```python
from build123d import *

# Parameters (mm, degrees)
SKETCH1_W           = 170
SKETCH1_H           = 145
BOSS_EXTRUDE1_DEPTH = 5
SKETCH2_W           = 150.6
SKETCH2_H           = 125.6
SKETCH2_W_2         = 144.4
SKETCH2_H_2         = 119.4
CUT_EXTRUDE1_DEPTH  = 2.5
SKETCH5_W           = 71
SKETCH5_H           = 7.5
SKETCH5_W_2         = 8
SKETCH5_H_2         = 25
BOSS_EXTRUDE2_DEPTH = 17.5
SKETCH6_W           = 2.5
SKETCH6_H           = 7.5
SKETCH6_H_2         = 25
BOSS_EXTRUDE3_DEPTH = 21.5
SKETCH7_W           = 71
SKETCH7_H           = 2.5
BOSS_EXTRUDE4_DEPTH = 4
BOSS_EXTRUDE6_DEPTH = 21.5


with BuildPart() as part:
    # Sketch1 → Boss-Extrude1 (new body)
    with BuildSketch(Plane(origin=(0, 0, 0), x_dir=(1, 0, 0), z_dir=(0, 1, 0))):
        Rectangle(SKETCH1_W, SKETCH1_H)
    extrude(amount=BOSS_EXTRUDE1_DEPTH)

    # Sketch2 → Cut-Extrude1 (cut)
    with BuildSketch(Plane(origin=(0, 5, 0), x_dir=(1, 0, 0), z_dir=(0, 1, 0))):
        Rectangle(SKETCH2_W, SKETCH2_H)
        Rectangle(SKETCH2_W_2, SKETCH2_H_2, mode=Mode.SUBTRACT)
    extrude(amount=-CUT_EXTRUDE1_DEPTH, mode=Mode.SUBTRACT)

    # Sketch5 → Boss-Extrude2 (add)
    with BuildSketch(Plane(origin=(0, 5, 0), x_dir=(1, 0, 0), z_dir=(0, 1, 0))):
        with Locations((0, 29.05)):
            Rectangle(SKETCH5_W, SKETCH5_H)
        with Locations((-31.5, -47.2)):
            Rectangle(SKETCH5_W_2, SKETCH5_H_2)
        with Locations((31.5, -47.2)):
            Rectangle(SKETCH5_W_2, SKETCH5_H_2)
    extrude(amount=BOSS_EXTRUDE2_DEPTH)

    # Sketch6 → Boss-Extrude3 (add)
    with BuildSketch(Plane(origin=(0, 5, 0), x_dir=(1, 0, 0), z_dir=(0, 1, 0))):
        with Locations((36.75, 29.05)):
            Rectangle(SKETCH6_W, SKETCH6_H)
        with Locations((-36.75, 29.05)):
            Rectangle(SKETCH6_W, SKETCH6_H)
        with Locations((36.75, -47.2)):
            Rectangle(SKETCH6_W, SKETCH6_H_2)
        with Locations((-36.75, -47.2)):
            Rectangle(SKETCH6_W, SKETCH6_H_2)
    extrude(amount=BOSS_EXTRUDE3_DEPTH)

    # Sketch7 → Boss-Extrude4 (add)
    with BuildSketch(Plane(origin=(0, 22.5, 0), x_dir=(1, 0, 0), z_dir=(0, 1, 0))):
        with Locations((0, 31.55)):
            Rectangle(SKETCH7_W, SKETCH7_H)
    extrude(amount=BOSS_EXTRUDE4_DEPTH)

    # Sketch9 → Boss-Extrude6 (add)
    with BuildSketch(Plane(origin=(0, 5, 0), x_dir=(1, 0, 0), z_dir=(0, 1, 0))):
        Polygon((38, -59.7), (72.2, -59.7), (72.2, -57.8), (72.2, 57.8), (72.2, 59.7), (-72.2, 59.7), (-72.2, 57.8), (-72.2, -57.8), (-72.2, -59.7), (-38, -59.7), (-38, -57.2), (-69.7, -57.8), (-69.7, 57.8), (69.7, 57.8), (69.7, -57.2), (38, -57.2), align=None)
    extrude(amount=BOSS_EXTRUDE6_DEPTH)


solid = part.part
```
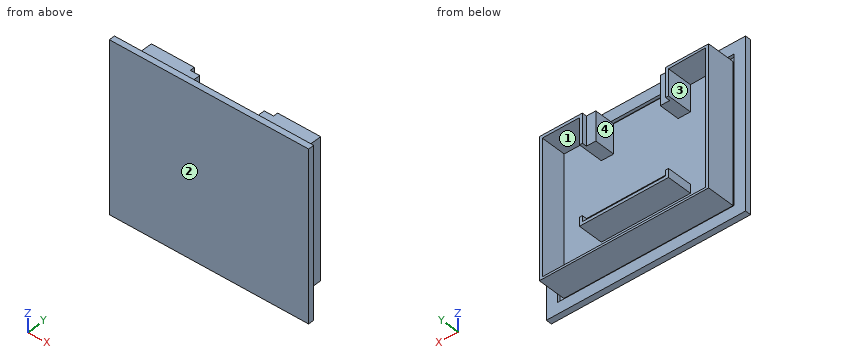
Check sheet for the modelled part. Datum: model origin and axes. Units: mm. Face numbers are marked on the shaded views. A direction names the side the tool comes from. Give positions to 0.01 mm unless a question says otherwise; leave off trailing zeros. Loops run counter-clockwise (first coordinate to the right, second up) from the corner with the lowest first, then second, coordinate; pieces in that order, holes last. Notation, with made-up numbers: (11, -21.5) - (32, -21.5) arc R21 ccw to (32, 3.5) - close; hole circle Ø11 at (-28.75, -11.75). An arc over 180 degrees is marked (long way). One line per question, with ' | ' between items. Start each with the question number.
1. Cross-section at A-A, the plane y = 18.25. Enter the section's corners in (x, z).
2. Material ranges on line 1 along Z through (x, y) = (-54.5, 2.75); line 2 along X through (y, z) = (5.5, 47); line 3 along Z through (x, y) = (14.5, 18.75), recorded low to high. Write a range as [from, to].
3. Cross-section at B-B, the plane z = 43.5. Enter the section's corners in (x, y).
4. Cross-section at D-D, the plane z = -52. Enter the section's corners in (x, y).
5. Cross-section at C-C, the plane x = 46.5. Enter the section's corners in (y, z), plus the area to 3 significant figures.
6. Draft check along Z on the marked faces 3 and 4. Enter one of: released by +Z, released by -Z, zero draft, split by the parting line, or undercut.
7. Gauge pin test, flat ends, axial feed: pin 1 Ø8 at (x, y) = (-12.5, 15) entering from +Z; pin 2 Ø14 at (y, z) = (13.5, 49) entering from -X; pin 3 Ø2 at (x, y) = (-11, 20.5) entering from -Z. Record the tip position at first contact, or that the pin passes through.
8. Set-up check for the marked faces 1 and 2: record each of +Z, -Z, +X, -X, +Y, -Y from which the full face is reachable in a straight line by a thin tool's end or side.
Check result:
1) outline: (-72.2, -59.7) - (72.2, -59.7) - (72.2, 59.7) - (27.5, 59.7) - (27.5, 34.7) - (38, 34.7) - (38, 57.2) - (69.7, 57.2) - (69.7, -57.8) - (-69.7, -57.8) - (-69.7, 57.8) - (-38, 57.2) - (-38, 34.7) - (-27.5, 34.7) - (-27.5, 59.7) - (-72.2, 59.7) - close; (-38, -32.8) - (38, -32.8) - (38, -25.3) - (-38, -25.3) - close
2) line 1: z = [-72.5, -62.8], [-59.7, 59.7], [62.8, 72.5] | line 2: x = [-72.2, -69.7], [-38, -27.5], [27.5, 38], [69.7, 72.2] | line 3: z = [-59.7, -57.8], [-32.8, -25.3]
3) outline: (-85, 0) - (85, 0) - (85, 5) - (75.3, 5) - (75.3, 2.5) - (72.2, 2.5) - (72.2, 26.5) - (69.7, 26.5) - (69.7, 5) - (38, 5) - (38, 26.5) - (35.5, 26.5) - (35.5, 22.5) - (27.5, 22.5) - (27.5, 5) - (-27.5, 5) - (-27.5, 22.5) - (-35.5, 22.5) - (-35.5, 26.5) - (-38, 26.5) - (-38, 5) - (-69.7, 5) - (-69.7, 26.5) - (-72.2, 26.5) - (-72.2, 2.5) - (-75.3, 2.5) - (-75.3, 5) - (-85, 5) - close
4) outline: (-85, 0) - (85, 0) - (85, 5) - (75.3, 5) - (75.3, 2.5) - (72.2, 2.5) - (72.2, 26.5) - (69.7, 26.5) - (69.7, 5) - (-69.7, 5) - (-69.7, 26.5) - (-72.2, 26.5) - (-72.2, 2.5) - (-75.3, 2.5) - (-75.3, 5) - (-85, 5) - close
5) outline: (0, -72.5) - (5, -72.5) - (5, -62.8) - (2.5, -62.8) - (2.5, -59.7) - (26.5, -59.7) - (26.5, -57.8) - (5, -57.8) - (5, 57.2) - (26.5, 57.2) - (26.5, 59.7) - (2.5, 59.7) - (2.5, 62.8) - (5, 62.8) - (5, 72.5) - (0, 72.5) - close | area: 804 mm2
6) face 3: undercut | face 4: zero draft
7) pin 1: stops at z = -25.3 | pin 2: stops at x = -72.2 | pin 3: stops at z = -59.7
8) face 1: +Y | face 2: +Z, -Z, +X, -X, -Y
